from build123d import *

# Parameters (mm, degrees)
FILLET1_R          = 2.54
SKETCH2_R          = 9.426821905
CUT_EXTRUDE1_DEPTH = 2.54


with BuildPart() as part:
    # Sketch1 → Revolve1 (revolve)
    with BuildSketch(Plane.XY):
        with BuildLine():
            Line((0, 0), (-38.1, 0))
            Line((-38.1, 0), (-38.1, 241.3))
            ThreePointArc((-38.1, 241.3), (-37.492793188, 243.708427101), (-35.816330275, 245.541100917))
            ThreePointArc((-35.816330275, 245.541100917), (-22.338916525, 251.83972175), (-7.62, 254))
            ThreePointArc((-7.62, 254), (-6.721974388, 254.371974388), (-6.35, 255.27))
            Line((-6.35, 255.27), (-6.35, 259.715))
            Line((-6.35, 259.715), (-12.7, 259.715))
            Line((-12.7, 259.715), (-12.7, 269.24))
            Line((-12.7, 269.24), (0, 269.24))
            Line((0, 269.24), (0, 0))
        make_face()
    revolve(axis=Axis((0, 0, 0), (0, 1, 0)))

    # Fillet1
    fillet1_edges = [part.edges().sort_by_distance(p)[0] for p in [
        (38.1, 0, 0),
    ]]
    fillet(fillet1_edges, radius=FILLET1_R)

    # Sketch2 → Cut-Extrude1 (cut)
    with BuildSketch(Plane(origin=(0, 269.24, 0), x_dir=(1, 0, 0), z_dir=(0, 1, 0))):
        Circle(SKETCH2_R)
    extrude(amount=-CUT_EXTRUDE1_DEPTH, mode=Mode.SUBTRACT)


solid = part.part
Model file for the job. Use its own axes, mm. A direction names the side the tool comes from. Give positions to 0.01 mm unless a question says otherwise; leave off trailing zeros. Loops run counter-clockwise (first coordinate to the right, second up) from the corner with the lowest first, then second, coordinate; pieces in that order, holes last. Notation, with made-up numbers: (34, -9.5) - (46, -9.5) arc R36 ccw to (46, 28.5) - close; hole circle Ø10 at (67, -35.5). An arc over 180 degrees is marked (long way). Use one line per item in the form item = value.
(1) Drop flat-ended pins along their axis: P1, Ø1.5, axis at y = 108.5, z = -17, coming from the +X side; P2, Ø10, axis at x = 18.5, z = -28, coming from the +Y side; P3, Ø1.5, axis at y = 180.5, z = 20, coming from the +X side. Give the stop position or say it passes through.
Determined:
P1 = 34.46
P2 = 249.52
P3 = 32.88
(2) Cut at A-A (y = 207). Give the cut face in (x, z), then the cut area to 3 significant figures.
Determined:
outline = circle Ø76.2 at (0, 0)
area = 4,560 mm^2
(3) Pull direction Z, two halves, no side cores. Call faces 3 (the face through (2.75, 264.54, -12.4)), 4 (the face through (0, 266.7, 0)), 5 (the face through (3, 259.715, 6)), 6 (the face through (9, 268, -2.8)): pulls with the +Z half, pulls with the -Z half, needs draft (parallel to the pull), parting line crosses it, or undercut.
Determined:
face_3 = parting line crosses it
face_4 = undercut
face_5 = needs draft
face_6 = undercut
(4) Drill centre lines: L1, parallel to Z at x = 0, y = 268.7; L2, parallel to Y at x = -4.5, z = -7.5 (3 decimals); L3, parallel to Y at x = -8.5, z = 8.5 (3 decimals). Where is each one in solid material? Low to high.
Determined:
L1 = -12.7 to -9.43, 9.43 to 12.7
L2 = 0 to 253.988, 259.715 to 266.7
L3 = 0 to 253.811, 259.715 to 269.24
(5) 3-axis set-ups, long thin cutter, end or side, ignore diameter. For faces 1 (the face through (1.9, 269.24, 9.5)), 2 (the face through (1.38, 257.52, -6.2)): which of +Z, -Z, +X, -X, +Y, -Y reach the whole face in a straight line?
Determined:
face_1 = +Z, -Z, +X, -X, +Y
face_2 = none
